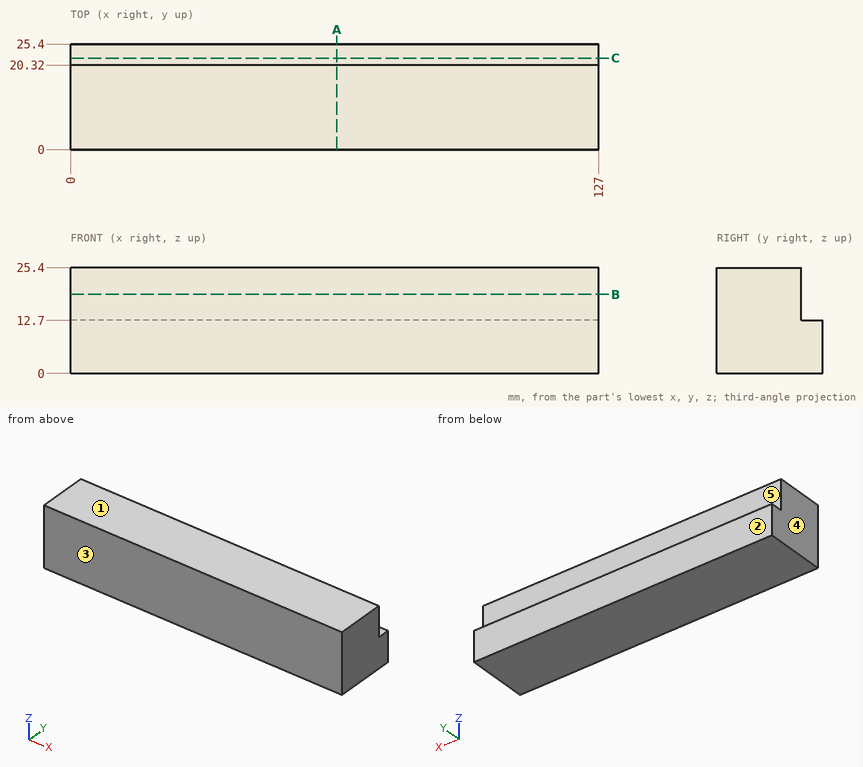
Can you work these out from the drawing? Everything is in mm from the part's minimum corner. A direction names the side the tool comes from. Give positions to 0.01 mm unless a question says otherwise; leave off trailing zeros. Loops run counter-clockwise (first coordinate to the right, second up) from the corner with the lowest first, then second, coordinate; pieces in that order, holes last. Notation, with made-up numbers: (75, 60) -> (130, 60) arc R24 ccw to (130, 77) -> close; hole circle Ø5 at (-8.5, 62.5). An arc over 180 degrees is marked (long way). Write item = value, one per line.
1) Will these pins go through, and if not, where does the flat tip stop? pin 1 (2.5 mm diameter, centred on x = 63.5, y = 23, fed in from +Z); pin 2 (14 mm diameter, centred on x = 62.5, z = 21.5, fed in from +Y).
Check result:
pin_1 = 12.7
pin_2 = 20.32
2) For the marked faces 4 and 5, which set-ups out of +Z, -Z, +X, -X, +Y, -Y let a thin tool reach every point of the face, with its end or its side?
Check result:
face_4 = +Z, -Z, -X, +Y, -Y
face_5 = +Z, +X, -X, +Y
3) Suppose I cut it at A-A on x = 64. Write out the boundary of the cut face in (y, z).
Check result:
outline = (0, 0) -> (25.4, 0) -> (25.4, 12.7) -> (20.32, 12.7) -> (20.32, 25.4) -> (0, 25.4) -> close
4) Thinking about a two-plate mould opening in Y: for the marked faces 1, 2 and 3, which applies, released by +Y, released by -Y, zero draft, split by the parting line, or undercut?
Check result:
face_1 = zero draft
face_2 = released by +Y
face_3 = released by -Y
5) Suppose I cut it at B-B on z = 19. Write out the boundary of the cut face in (x, y).
Check result:
outline = (0, 0) -> (127, 0) -> (127, 20.32) -> (0, 20.32) -> close
6) I need wall thicknesses on L1, parallel to Y at x = 92.5, z = 20; L2, parallel to Z at x = 26.5, y = 23. Which ranges of each line are inside material? Lowest first, please. Write a range as from..to.
Check result:
L1 = 0..20.32
L2 = 0..12.7
7) Suppose I cut it at C-C on y = 22. Write out the boundary of the cut face in (x, z), then the cut area to 3 significant figures.
Check result:
outline = (0, 0) -> (127, 0) -> (127, 12.7) -> (0, 12.7) -> close
area = 1,610 mm2
